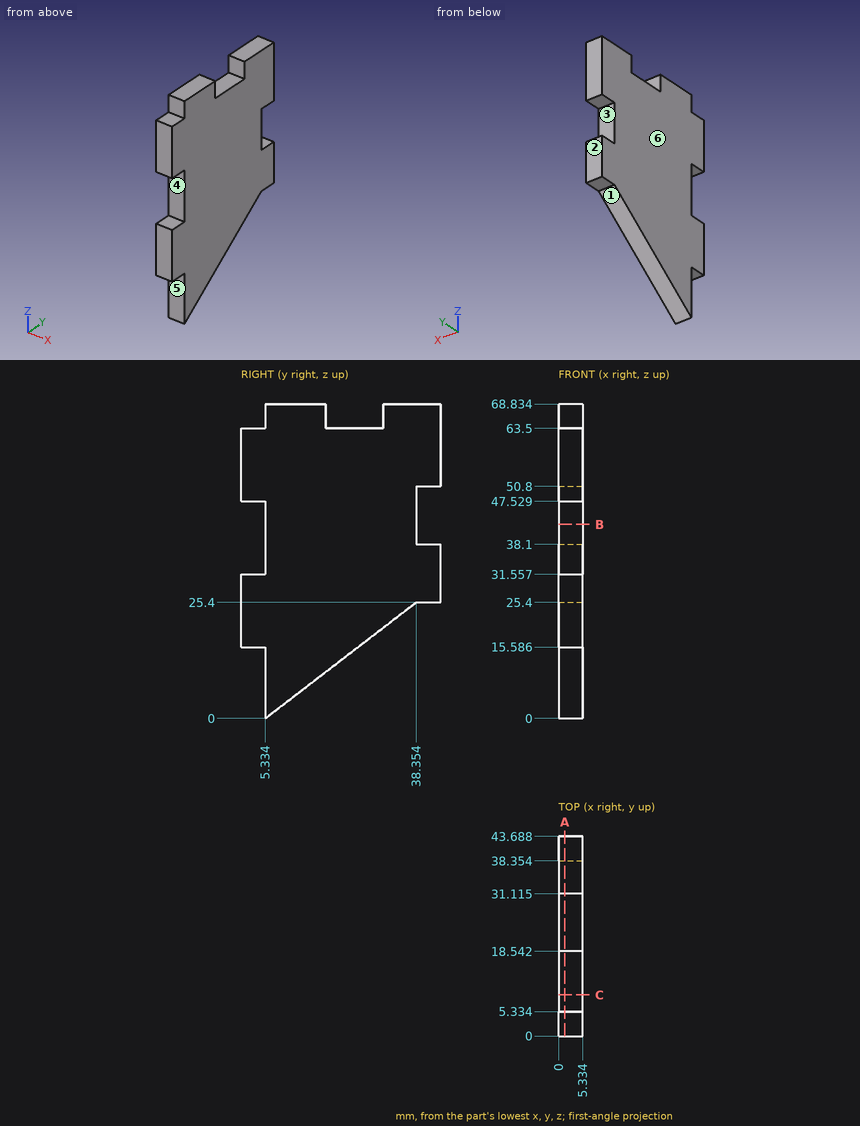
Here's the drawing with two shaded views (mm, measured from the low corner). I have some questions. A direction names the side the tool comes from. Give positions to 0.01 mm unless a question says otherwise; leave off trailing zeros. Loops run counter-clockwise (first coordinate to the right, second up) from the corner with the lowest first, then second, coordinate; pieces in that order, holes last. Notation, with made-up numbers: (69.5, 19.25) - (108.5, 19.25) arc R7 cw to (108.5, 25.25) - close; hole circle Ø11 at (26.5, 14). An arc over 180 degrees is marked (long way). Answer in a Markdown table with one row per item. Add a question column.
Q1. If we section it at B-B (z = 42.5): List the corners of the cut face in (x, y) for me.
Q2. If we section it at C-C (y = 9): List the corners of the cut face in (x, z) for me, plus the area to 3 significant figures.
Q3. Which directions (+Z, -Z, +X, -X, +Y, -Y) give clear straight access to the entire face, cutting with the end or side of a thin tool? Please do the marked faces 4, 5 and 6.
Q4. If we section it at A-A (x = 1.35): List the corners of the cut face in (y, z) for me (1 decimal), plus the area to 3 significant figures.
Q5. Please list where these lines run through material, in increasing order: L1, parallel to Z at x = 2.9, y = 5; L2, parallel to Y at x = 3.55, z = 35.5; L3, parallel to Y at x = 3.9, z = 38.5. Write a range as from..to.
Q6. For pin 1 (1.6 mm diameter, centred on x = 2, y = 3, fed in from +Z); pin 2 (2.5 mm diameter, centred on x = 2.5, z = 67.5, fed in from -Y); pin 3 (1.6 mm diameter, centred on x = 4, y = 40, fed in from -Z), each with a flat end and sliding along its axis, tell me the tip position at first contact or that it passes through.
Q7. We'd pull the mould along Z, two halves only. Please class the marked faces 1, 2 and 3: +Z half, -Z half, draft (parallel to the pull), parting line (faces both ways), or undercut.
The answers:
| question | item | result |
|---|---|---|
| 1 | outline | (0, 5.33) - (5.33, 5.33) - (5.33, 38.35) - (0, 38.35) - close |
| 2 | outline | (0, 2.82) - (5.33, 2.82) - (5.33, 68.83) - (0, 68.83) - close |
| 2 | area | 352 mm^2 |
| 3 | face 4 | +X, -X, -Y |
| 3 | face 5 | -Z, +X, -X, -Y |
| 3 | face 6 | +Z, -Z, -X, +Y, -Y |
| 4 | outline | (0, 15.6) - (5.3, 15.6) - (5.3, 0) - (38.4, 25.4) - (43.7, 25.4) - (43.7, 38.1) - (38.4, 38.1) - (38.4, 50.8) - (43.7, 50.8) - (43.7, 68.8) - (31.1, 68.8) - (31.1, 63.5) - (18.5, 63.5) - (18.5, 68.8) - (5.3, 68.8) - (5.3, 63.5) - (0, 63.5) - (0, 47.5) - (5.3, 47.5) - (5.3, 31.6) - (0, 31.6) - close |
| 4 | area | 2,120 mm^2 |
| 5 | L1 | z = 15.59..31.56, 47.53..63.5 |
| 5 | L2 | y = 5.33..43.69 |
| 5 | L3 | y = 5.33..38.35 |
| 6 | pin 1 | stops at z = 63.5 |
| 6 | pin 2 | stops at y = 5.33 |
| 6 | pin 3 | stops at z = 25.4 |
| 7 | face 1 | -Z half |
| 7 | face 2 | draft |
| 7 | face 3 | undercut |
